Autodesk Inventor part; units mm, degrees
ref_plane "YZ Plane" through (0, 0, 0) normal (1, 0, 0) x (0, 1, 0)
ref_plane "XZ Plane" through (0, 0, 0) normal (0, 1, 0) x (-1, 0, 0)
ref_plane "XY Plane" through (0, 0, 0) normal (0, 0, 1) x (1, 0, 0)
sketch "Sketch1" plane through (0, 0, 0) normal (0, 0, 1) x (1, 0, 0)
  circle A0 centre (0, 0) radius 5.85 construction
  circle A1 centre (0, 0) radius 2.95 construction
  circle A2 centre (0, 0) radius 3.1
  circle A3 centre (0, 0) radius 8
  dimension "d0" = 11.7
  dimension "d1" = 5.9
  dimension "d2" = 6.2
  dimension "d3" = 16
extrude "Extrusion1" add sketch "Sketch1" along normal blind 3 contours A2 | A3
sketch "Sketch2" plane through (0, 0, 3) normal (0, 0, 1) x (1, 0, 0)
  circle A0 centre (0, 0) radius 4.935 construction
  circle A1 centre (0, 0) radius 2.95 construction
  circle A2 centre (0, 0) radius 8
  circle A3 centre (0, 0) radius 5.25
  dimension "d6" = 9.87
  dimension "d7" = 5.9
  dimension "d10" = 10.5
extrude "Extrusion2" add sketch "Sketch2" along normal blind 4
sketch "Sketch3" plane through (0, 0, 0) normal (0, 0, -1) x (-1, 0, 0)
  circle A0 centre (0, 0) radius 8 construction
  circle A1 centre (0, 1.755) radius 3.1
  circle A2 centre (0, 0) radius 8 construction
  line L0 (0, -11.2) -> (0, 11.2) construction
  circle A3 centre (0, -2.095) radius 1.5 construction
  circle A4 centre (0, 1.755) radius 1.5 construction
  circle A5 centre (0, 0) radius 4.855 construction
  dimension "d13" = 6.2
  dimension "d14" = 3
  dimension "d15" = 3
  dimension "d16" = 3.85
  dimension "d21" = 9.71
  dimension "d22" = 1.6
extrude "Extrusion3" cut sketch "Sketch3" against normal through all
properties part number "30_raspi_lens_to_laser"
Geometry check sheet. Reference: the model listing, model coordinates, mm. A direction names the side the tool comes from. Give positions to 0.01 mm unless a question says otherwise; leave off trailing zeros. Order: outer loops, then holes, each group sorted by start corner. A loop starts at its lowest first (then second) coordinate and runs counter-clockwise, first axis right, second up. Notation, with made-up numbers: (-19, 62.25) - (11, 62.25) arc R21 ccw to (11, 87.25) - close; hole circle Ø7 at (89, 21). An arc over 180 degrees is marked (long way). Answer as a JSON object with one key per item and string values.
(1) Cross-section at A-A (x = 0). Record the cut outline in (y, z) (3 decimals).
Report:
{"outline": "(-8, 0) - (-1.345, 0) - (-1.345, 3) - (-5.25, 3) - (-5.25, 7) - (-8, 7) - close; (4.855, 0) - (8, 0) - (8, 7) - (5.25, 7) - (5.25, 3) - (4.855, 3) - close"}
(2) Cross-section at C-C (z = 5.75). Record the cut outline in (x, y).
Report:
{"outline": "circle Ø16 at (0, 0); hole circle Ø10.5 at (0, 0)"}
(3) Material ranges on line 1 (Y direction, x = 0, z = 0.65) (3 decimals); line 2 (Z direction, x = 3.5, y = 3.5); line 3 (Y direction, x = 0, z = 6.1), recorded low to high.
Report:
{"line 1": "-8 to -1.345, 4.855 to 8", "line 2": "0 to 3", "line 3": "-8 to -5.25, 5.25 to 8"}
(4) Cross-section at B-B (y = 0.75). Record the cut outline in (x, z).
Report:
{"outline": "(-7.96, 0) - (-2.93, 0) - (-2.93, 3) - (-5.2, 3) - (-5.2, 7) - (-7.96, 7) - close; (2.93, 0) - (7.96, 0) - (7.96, 7) - (5.2, 7) - (5.2, 3) - (2.93, 3) - close"}
(5) Draft check along Y on faces 3 (the cylindrical face through (-2.957, 2.686, 1.479)), 4 (the flat face through (5.2, -1.7, 7)), 5 (the cylindrical face through (-1.73, 7.81, 3.45)). Enter one of: released by +Y, released by -Y, zero draft, split by the parting line, or undercut.
Report:
{"face 3": "undercut", "face 4": "zero draft", "face 5": "split by the parting line"}
(6) Depth check by flat-ended pin: pin 1 Ø1.5 at (x, z) = (3, 6) entering from +Y; pin 2 Ø2 at (x, z) = (-6, 1.5) entering from +Y (3 decimals); pin 3 Ø1.5 at (y, z) = (3.5, 3) entering from -X. Enter the tip coordinate at first touch or a pass-through.
Report:
{"pin 1": "y = 7.68", "pin 2": "y = 6.245", "pin 3": "x = -7.51"}
(7) Tool access check on faces 1 (the flat face through (0, -2, 0)), 2 (the flat face through (0, -2, 3)). Record the directions out of +Z, -Z, +X, -X, +Y, -Y that give a thin tool (end or side, any length) a straight path to the whole face; none if there is none.
Report:
{"face 1": "-Z, +X, -X, +Y, -Y", "face 2": "+Z"}
(8) Cross-section at D-D (x = -4.75). Record the cut outline in (y, z), then the cut area to 3 significant figures.
Report:
{"outline": "(-6.44, 0) - (6.44, 0) - (6.44, 7) - (2.24, 7) - (2.24, 3) - (-2.24, 3) - (-2.24, 7) - (-6.44, 7) - close", "area": "72.2 mm^2"}
